```python
from build123d import *

# Parameters (mm, degrees)
SKETCH2_W           = 150
SKETCH2_H           = 80
SKETCH2_R           = 1.5
BOSS_EXTRUDE1_DEPTH = 3
SKETCH5_R           = 5
SKETCH5_R_2         = 2.5
BOSS_EXTRUDE3_DEPTH = 70
SKETCH7_R           = 1.5
CUT_EXTRUDE1_DEPTH  = 10
SKETCH3_R           = 2.25
CUT_EXTRUDE2_DEPTH  = 5


with BuildPart() as part:
    # Sketch2 → Boss-Extrude1 (new body)
    with BuildSketch(Plane(origin=(0, 0, 0), x_dir=(1, 0, 0), z_dir=(0, 1, 0))):
        with Locations((-8.46473029, 1.825726141)):
            Rectangle(SKETCH2_W, SKETCH2_H)
        with Locations((-68.46473029, 11.325726141)):
            Circle(SKETCH2_R, mode=Mode.SUBTRACT)
        with Locations((-68.46473029, -7.674273859)):
            Circle(SKETCH2_R, mode=Mode.SUBTRACT)
        with Locations((-76.46473029, 11.325726141)):
            Circle(SKETCH2_R, mode=Mode.SUBTRACT)
        with Locations((-76.46473029, -7.674273859)):
            Circle(SKETCH2_R, mode=Mode.SUBTRACT)
        with Locations((51.53526971, -7.674273859)):
            Circle(SKETCH2_R, mode=Mode.SUBTRACT)
        with Locations((59.53526971, -7.674273859)):
            Circle(SKETCH2_R, mode=Mode.SUBTRACT)
        with Locations((59.53526971, 11.325726141)):
            Circle(SKETCH2_R, mode=Mode.SUBTRACT)
        with Locations((51.53526971, 11.325726141)):
            Circle(SKETCH2_R, mode=Mode.SUBTRACT)
    extrude(amount=-BOSS_EXTRUDE1_DEPTH)

    # Sketch5 → Boss-Extrude3 (add)
    with BuildSketch(Plane.XZ.offset(3)):
        with Locations((-73.46473029, 28.174273859)):
            Circle(SKETCH5_R)
        with Locations((-73.46473029, 28.174273859)):
            Circle(SKETCH5_R_2, mode=Mode.SUBTRACT)
        with Locations((56.53526971, 28.174273859)):
            Circle(SKETCH5_R)
        with Locations((56.53526971, 28.174273859)):
            Circle(SKETCH5_R_2, mode=Mode.SUBTRACT)
        with Locations((56.53526971, -31.825726141)):
            Circle(SKETCH5_R)
        with Locations((56.53526971, -31.825726141)):
            Circle(SKETCH5_R_2, mode=Mode.SUBTRACT)
        with Locations((-73.46473029, -31.825726141)):
            Circle(SKETCH5_R)
        with Locations((-73.46473029, -31.825726141)):
            Circle(SKETCH5_R_2, mode=Mode.SUBTRACT)
    extrude(amount=BOSS_EXTRUDE3_DEPTH)

    # Sketch7 → Cut-Extrude1 (cut)
    with BuildSketch(Plane(origin=(0, 0, 0), x_dir=(1, 0, 0), z_dir=(0, 1, 0))):
        with Locations((-56.449797454, 34.724662311)):
            Circle(SKETCH7_R)
        with Locations((-56.449797454, 19.620815473)):
            Circle(SKETCH7_R)
        with Locations((39.655256431, 34.724662311)):
            Circle(SKETCH7_R)
        with Locations((39.655256431, 19.620815473)):
            Circle(SKETCH7_R)
        with Locations((-56.284289699, -15.969363191)):
            Circle(SKETCH7_R)
        with Locations((-56.284289699, -31.073210029)):
            Circle(SKETCH7_R)
        with Locations((39.820764186, -15.969363191)):
            Circle(SKETCH7_R)
        with Locations((39.820764186, -31.073210029)):
            Circle(SKETCH7_R)
    extrude(amount=-CUT_EXTRUDE1_DEPTH, mode=Mode.SUBTRACT)

    # Sketch3 → Cut-Extrude2 (cut)
    with BuildSketch(Plane(origin=(0, 0, 0), x_dir=(1, 0, 0), z_dir=(0, 1, 0))):
        with Locations((56.53526971, 31.825726141)):
            Circle(SKETCH3_R)
        with Locations((56.53526971, -28.174273859)):
            Circle(SKETCH3_R)
        with Locations((-73.46473029, -28.174273859)):
            Circle(SKETCH3_R)
        with Locations((-73.46473029, 31.825726141)):
            Circle(SKETCH3_R)
    extrude(amount=-CUT_EXTRUDE2_DEPTH, mode=Mode.SUBTRACT)


solid = part.part
```
Source: CAD feature listing. Evaluate the final solid. Frame: model axes, mm. A direction names the side the tool comes from. Round coordinates to 2 decimals unless told otherwise and drop trailing zeros. Loops run counter-clockwise (first coordinate to the right, second up) from the corner with the lowest first, then second, coordinate; pieces in that order, holes last. Notation, with made-up numbers: (3, 59.25) - (29, 59.25) arc R22 cw to (29, 94.25) - close; hole circle Ø6 at (-20.5, -9). An arc over 180 degrees is marked (long way). Use CSV: the item, a comma, the result in double quotes.
Q1. Section query B-B, the plane x = 45.5. Output: boundary loops of the cut face in (y, z), then the cut area to 3 significant figures.
Reported:
outline,"(-3, -41.83) - (0, -41.83) - (0, 38.17) - (-3, 38.17) - close"
area,"240 mm^2"
Q2. Ray query, line 1 along Z through (x, y) = (-73, -60.5); line 2 along Z through (x, y) = (55, -41); line 3 along Y through (x, z) = (-25, 25). Return the intervals inside material, ascending.
Reported:
line 1,"-36.8 to -34.28, -29.37 to -26.85, 23.2 to 25.72, 30.63 to 33.15"
line 2,"-36.58 to -33.8, -29.85 to -27.07, 23.42 to 26.2, 30.15 to 32.93"
line 3,"-3 to 0"
Q3. Mould query, pull axis Z, two halves, no side actions, for faces 1 (the flat face through (-10, -1, 38.174)), 2 (the cylindrical face through (38.55, -1.48, -35.74)), 3 (the flat face through (54, -73, 27)). Classes: pulls with the +Z half, pulls with the -Z half, needs draft (parallel to the pull), parting line crosses it, or undercut.
Reported:
face 1,"pulls with the +Z half"
face 2,"undercut"
face 3,"needs draft"
Q4. Reachability of faces 4 (the cylindrical face through (-75.31, -37.51, 29.86)), 5 (the cylindrical face through (60.966, -1.479, 7.224)) from +Z, -Z, +X, -X, +Y, -Y: full face, straight path, thin tool, end or side. Return the list, or none.
Reported:
face 4,"-Y"
face 5,"+Y, -Y"
Q5. Section query A-A, the plane y = -35. Output: boundary loops of the cut face in (x, z).
Reported:
outline,"circle Ø10 at (-73.46, -31.83); circle Ø10 at (-73.46, 28.17); circle Ø10 at (56.54, -31.83); circle Ø10 at (56.54, 28.17); hole circle Ø5 at (-73.46, -31.83); hole circle Ø5 at (-73.46, 28.17); hole circle Ø5 at (56.54, -31.83); hole circle Ø5 at (56.54, 28.17)"
Q6. Pin query (flat end, axial travel): pin 1 Ø6 at (x, z) = (21, -18) entering from -Y; pin 2 Ø1 at (y, z) = (-63.5, 29) entering from -X. Return the tip coordinate at first contact, or that it passes through.
Reported:
pin 1,"y = -3"
pin 2,"x = -78.45"
Q7. Section query C-C, the plane z = -3. Output: boundary loops of the cut face in (x, y), then the cut area to 3 significant figures.
Reported:
outline,"(-83.46, -3) - (66.54, -3) - (66.54, 0) - (-83.46, 0) - close"
area,"450 mm^2"
